Work out the finished part from the listing and answer in its coordinate system (mm). Face numbers are marked on the shaded views. A direction names the side the tool comes from. Round coordinates to 2 decimals unless told otherwise and drop trailing zeros. Order: outer loops, then holes, each group sorted by start corner. A loop starts at its lowest first (then second) coordinate and runs counter-clockwise, first axis right, second up. Notation, with made-up numbers: (58, 14.25) - (98, 14.25) arc R14 cw to (98, 41.25) - close; hole circle Ø1 at (-36.5, 42). An arc over 180 degrees is marked (long way). Answer in a Markdown table with one row per item.
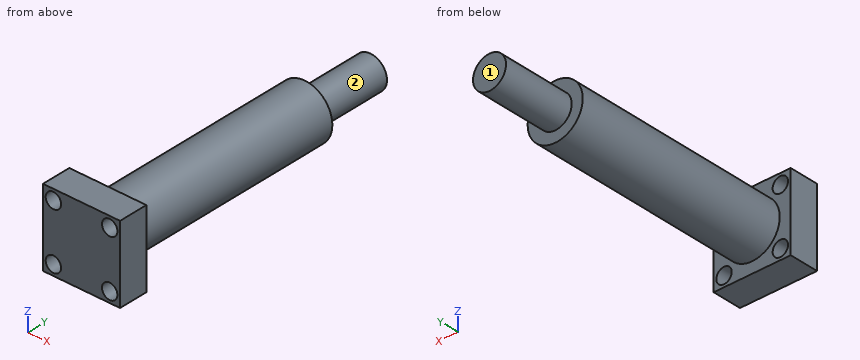
from build123d import *

# Parameters (mm, degrees)
SKETCH_1_R      = 7.5
EXTRUDE_1_DEPTH = 68
SKETCH_2_W      = 21
SKETCH_2_H      = 21
SKETCH_2_R      = 2.1
EXTRUDE_2_DEPTH = 8
SKETCH_3_R      = 4.5
EXTRUDE_3_DEPTH = 20


with BuildPart() as part:
    # 草图1 → 凸台-拉伸1 (new body)
    with BuildSketch(Plane(origin=(0, 0, 0), x_dir=(1, 0, 0), z_dir=(0, 1, 0))):
        with Locations(Location((0, 0, 0), (0, 0, 270))):
            Circle(SKETCH_1_R)
    extrude(amount=EXTRUDE_1_DEPTH)

    # 草图2 → 凸台-拉伸2 (add)
    with BuildSketch(Plane.XZ):
        Rectangle(SKETCH_2_W, SKETCH_2_H)
        with Locations(Location((-7.671572875, 7.671572875, 0), (0, 0, 270))):
            Circle(SKETCH_2_R, mode=Mode.SUBTRACT)
        with Locations(Location((7.671572875, -7.671572875, 0), (0, 0, 270))):
            Circle(SKETCH_2_R, mode=Mode.SUBTRACT)
        with Locations(Location((7.671572875, 7.671572875, 0), (0, 0, 270))):
            Circle(SKETCH_2_R, mode=Mode.SUBTRACT)
        with Locations(Location((-7.671572875, -7.671572875, 0), (0, 0, 270))):
            Circle(SKETCH_2_R, mode=Mode.SUBTRACT)
    extrude(amount=-EXTRUDE_2_DEPTH)

    # 草图3 → 凸台-拉伸3 (add)
    with BuildSketch(Plane(origin=(0, 68, 0), x_dir=(1, 0, 0), z_dir=(0, 1, 0))):
        with Locations(Location((0, 0, 0), (0, 0, 270))):
            Circle(SKETCH_3_R)
    extrude(amount=EXTRUDE_3_DEPTH)


solid = part.part
1) Find section D-D, the plane y = 27. Give the vertices of the cut face in (x, z), then the cut area to 3 significant figures.
Filled in:
| item | result |
|---|---|
| outline | circle Ø15 at (0, 0) |
| area | 177 mm^2 |
2) Find section B-B, the plane x = 0. Give the vertices of the cut face in (y, z), then the cut area to 3 significant figures.
Filled in:
| item | result |
|---|---|
| outline | (0, -10.5) - (8, -10.5) - (8, -7.5) - (68, -7.5) - (68, -4.5) - (88, -4.5) - (88, 4.5) - (68, 4.5) - (68, 7.5) - (8, 7.5) - (8, 10.5) - (0, 10.5) - close |
| area | 1,250 mm^2 |
3) Each of these flat-tipped pins is pushed along its axis until it touches: pin 1 (3 mm diameter, centred on y = 63, z = 0.5, fed in from -X); pin 2 (1 mm diameter, centred on x = 7.5, z = -5.5, fed in from +Y); pin 3 (1 mm diameter, centred on y = 64, z = 5, fed in from -X). Where does it stop, or does it pass through?
Filled in:
| item | result |
|---|---|
| pin 1 | stops at x = -7.5 |
| pin 2 | stops at y = 8 |
| pin 3 | stops at x = -6 |
4) Find the intervals of material crossed by probe 1 along Z at (x, y) = (-0.25, 69); probe 2 along Y at (x, z) = (-0.5, 8.75); probe 3 along X at (y, z) = (45.5, 0.5), in increasing order. Write a range as from..to.
Filled in:
| item | result |
|---|---|
| probe 1 | z = -4.49..4.49 |
| probe 2 | y = 0..8 |
| probe 3 | x = -7.48..7.48 |
5) Which of the six approach directions +Z, -Z, +X, -X, +Y, -Y give full straight-line access (tool end or side, diameter ignored) to the marked faces 1 and 2?
Filled in:
| item | result |
|---|---|
| face 1 | +Z, -Z, +X, -X, +Y |
| face 2 | +Y |
6) Find section C-C, the plane z = 8.5. Give the vertices of the cut face in (x, y).
Filled in:
| item | result |
|---|---|
| outline | (-10.5, 0) - (-9.6, 0) - (-9.6, 8) - (-10.5, 8) - close; (-5.74, 0) - (5.74, 0) - (5.74, 8) - (-5.74, 8) - close; (9.6, 0) - (10.5, 0) - (10.5, 8) - (9.6, 8) - close |
7) Find section A-A, the plane z = 0. Give the vertices of the cut face in (x, y), then the cut area to 3 significant figures.
Filled in:
| item | result |
|---|---|
| outline | (-10.5, 0) - (10.5, 0) - (10.5, 8) - (7.5, 8) - (7.5, 68) - (4.5, 68) - (4.5, 88) - (-4.5, 88) - (-4.5, 68) - (-7.5, 68) - (-7.5, 8) - (-10.5, 8) - close |
| area | 1,250 mm^2 |
